Read the model definition and answer for the solid it produces. Units are mm, in the model's axes. Face numbers are marked on the shaded views. A direction names the side the tool comes from. Round coordinates to 2 decimals unless told otherwise and drop trailing zeros. Loops run counter-clockwise (first coordinate to the right, second up) from the corner with the lowest first, then second, coordinate; pieces in that order, holes last. Notation, with made-up numbers: M 50,52.25 L 76,52.25 A18 cw 76,78.25 Z; hole C 59,-27.5 d8. An arc over 180 degrees is marked long. Write each question's results on one line, items separated by ' | '.
from build123d import *
from OCP.BRepFilletAPI import BRepFilletAPI_MakeChamfer

# Parameters (mm, degrees)
ESQUISSE1_W             = 20
ESQUISSE1_H             = 34
BOSS_EXTRU_1_DEPTH      = 4
ESQUISSE2_W             = 8
ESQUISSE2_H             = 7
ENL_V_MAT_EXTRU_1_DEPTH = 21.124611797
CONG_1_R                = 4
ESQUISSE3_W             = 6
ESQUISSE3_H             = 34
BOSS_EXTRU_2_DEPTH      = 20
ESQUISSE4_R             = 2.1
ENL_V_MAT_EXTRU_2_DEPTH = 36.566838488
CHANFREIN1_SIZE         = 8
CHANFREIN1_SIZE2        = 4.618802154
CONG_2_R                = 4
ESQUISSE5_R             = 3.2
ENL_V_MAT_EXTRU_3_DEPTH = 29.08914381
ESQUISSE6_R             = 5.5
ENL_V_MAT_EXTRU_4_DEPTH = 29.08914381
ENL_V_MAT_EXTRU_5_DEPTH = 36.566838488
CONG_3_R                = 4
ESQUISSE9_W             = 30.59391243
ESQUISSE9_H             = 32.996523038
ENL_V_MAT_EXTRU_6_DEPTH = 1
ESQUISSE10_R            = 4
ENL_V_MAT_EXTRU_7_DEPTH = 3


with BuildPart() as part:
    # Esquisse1 → Boss.-Extru.1 (new body)
    with BuildSketch(Plane.XY):
        Rectangle(ESQUISSE1_W, ESQUISSE1_H)
    extrude(amount=BOSS_EXTRU_1_DEPTH)

    # Esquisse2 → Enlèv. mat.-Extru.1 (cut, through all)
    with BuildSketch(Plane.XY.offset(4)):
        with Locations((0, 13.5)):
            Rectangle(ESQUISSE2_W, ESQUISSE2_H)
        with Locations((0, -13.5)):
            Rectangle(ESQUISSE2_W, ESQUISSE2_H)
    extrude(amount=-ENL_V_MAT_EXTRU_1_DEPTH, mode=Mode.SUBTRACT)

    # Congé1
    cong_1_edges = [part.edges().sort_by_distance(p)[0] for p in [
        (0, -10, 4),
        (0, 10, 4),
    ]]
    fillet(cong_1_edges, radius=CONG_1_R - 0.0001)  # a hair under: the kernel refuses the full size

    # Esquisse3 → Boss.-Extru.2 (add)
    with BuildSketch(Plane.XY.offset(4)):
        with Locations((-7, 0)):
            Rectangle(ESQUISSE3_W, ESQUISSE3_H)
        with Locations((7, 0)):
            Rectangle(ESQUISSE3_W, ESQUISSE3_H)
    extrude(amount=BOSS_EXTRU_2_DEPTH)

    # Esquisse4 → Enlèv. mat.-Extru.2 (cut, through all)
    with BuildSketch(Plane(origin=(10, 0, 0), x_dir=(0, 0, -1), z_dir=(1, 0, 0))):
        with Locations(Location((-19, 9, 0), (0, 0, 90))):
            Circle(ESQUISSE4_R)
        with Locations(Location((-19, -9, 0), (0, 0, 90))):
            Circle(ESQUISSE4_R)
    extrude(amount=-ENL_V_MAT_EXTRU_2_DEPTH, mode=Mode.SUBTRACT)

    # Chanfrein1: one chamfer whose edges measure the first distance from different faces: ONE call of the kernel's chamfer builder (chamfer() names one face for all edges)
    chanfrein1_edges_1 = [part.edges().sort_by_distance(p)[0] for p in [
        (-7, -17, 24),
    ]]
    chanfrein1_side_1 = [part.faces().sort_by_distance(p)[0] for p in [
        (-7, -17, 12),
    ]]
    chanfrein1_edges_2 = [part.edges().sort_by_distance(p)[0] for p in [
        (-7, 17, 24),
    ]]
    chanfrein1_side_2 = [part.faces().sort_by_distance(p)[0] for p in [
        (-7, 17, 12),
    ]]
    chanfrein1_edges_3 = [part.edges().sort_by_distance(p)[0] for p in [
        (7, -17, 24),
    ]]
    chanfrein1_side_3 = [part.faces().sort_by_distance(p)[0] for p in [
        (7, -17, 12),
    ]]
    chanfrein1_edges_4 = [part.edges().sort_by_distance(p)[0] for p in [
        (7, 17, 24),
    ]]
    chanfrein1_side_4 = [part.faces().sort_by_distance(p)[0] for p in [
        (7, 17, 12),
    ]]
    chanfrein1 = BRepFilletAPI_MakeChamfer(part.part.solid().wrapped)
    for e in chanfrein1_edges_1:
        chanfrein1.Add(CHANFREIN1_SIZE, CHANFREIN1_SIZE2, e.wrapped, chanfrein1_side_1[0].wrapped)  # the first distance lies on this face
    for e in chanfrein1_edges_2:
        chanfrein1.Add(CHANFREIN1_SIZE, CHANFREIN1_SIZE2, e.wrapped, chanfrein1_side_2[0].wrapped)  # the first distance lies on this face
    for e in chanfrein1_edges_3:
        chanfrein1.Add(CHANFREIN1_SIZE, CHANFREIN1_SIZE2, e.wrapped, chanfrein1_side_3[0].wrapped)  # the first distance lies on this face
    for e in chanfrein1_edges_4:
        chanfrein1.Add(CHANFREIN1_SIZE, CHANFREIN1_SIZE2, e.wrapped, chanfrein1_side_4[0].wrapped)  # the first distance lies on this face
    add(Compound.cast(chanfrein1.Shape()), mode=Mode.REPLACE)

    # Congé2
    cong_2_edges = [part.edges().sort_by_distance(p)[0] for p in [
        (-7, 12.381197846, 24),
        (-7, -12.381197846, 24),
        (-7, -17, 16),
        (7, 12.381197846, 24),
        (7, -12.381197846, 24),
        (7, -17, 16),
        (-7, 17, 16),
        (7, 17, 16),
    ]]
    fillet(cong_2_edges, radius=CONG_2_R)

    # Esquisse5 → Enlèv. mat.-Extru.3 (cut, through all)
    with BuildSketch(Plane.XY.offset(4)):
        Circle(ESQUISSE5_R)
    extrude(amount=-ENL_V_MAT_EXTRU_3_DEPTH, mode=Mode.SUBTRACT)

    # Esquisse6 → Enlèv. mat.-Extru.4 (cut, through all)
    with BuildSketch(Plane.XY.offset(4)):
        Circle(ESQUISSE6_R)
    extrude(amount=ENL_V_MAT_EXTRU_4_DEPTH, mode=Mode.SUBTRACT)

    # Esquisse8 → Enlèv. mat.-Extru.5 (cut, through all)
    with BuildSketch(Plane(origin=(10, 0, 0), x_dir=(0, 0, -1), z_dir=(1, 0, 0))):
        Polygon((0, 17), (0, 10), (-24, -3), (-24, 17), align=None)
    extrude(amount=-ENL_V_MAT_EXTRU_5_DEPTH, mode=Mode.SUBTRACT)

    # Congé3
    cong_3_edges = [part.edges().sort_by_distance(p)[0] for p in [
        (7.304886114, -3, 24),
        (-7.304886114, -3, 24),
    ]]
    fillet(cong_3_edges, radius=CONG_3_R)

    # Esquisse9 → Enlèv. mat.-Extru.6 (cut)
    with BuildSketch(Plane(origin=(10, 0, 0), x_dir=(0, 0, -1), z_dir=(1, 0, 0))):
        with Locations((-11.472185, -1.799431883)):
            Rectangle(ESQUISSE9_W, ESQUISSE9_H)
    extrude(amount=-ENL_V_MAT_EXTRU_6_DEPTH, mode=Mode.SUBTRACT)

    # Esquisse10 → Enlèv. mat.-Extru.7 (cut)
    with BuildSketch(Plane(origin=(9, 0, 0), x_dir=(0, 0, -1), z_dir=(1, 0, 0))):
        with Locations(Location((-19, -9, 0), (0, 0, 90))):
            Circle(ESQUISSE10_R)
    extrude(amount=-ENL_V_MAT_EXTRU_7_DEPTH, mode=Mode.SUBTRACT)


solid = part.part
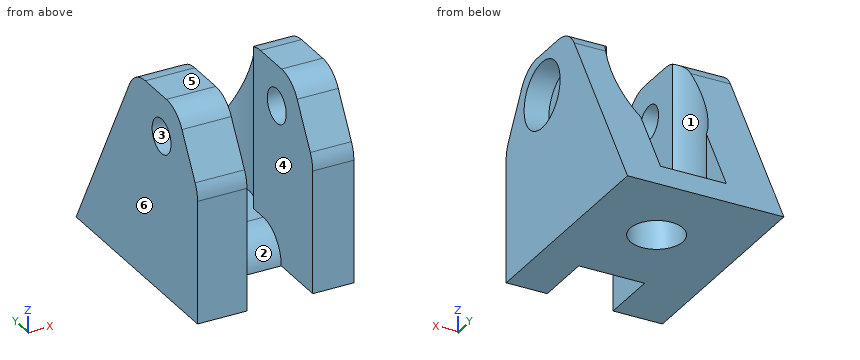
Item 1: The part is cut by section D-D (x = -7.75). Determine the outline of the cut face in (y, z).
Outcome:
outline: M -17,0 L 10,0 L -1.87,21.91 A4 ccw -5.38,24 L -10.07,24 A4 ccw -13.54,22 L -16.46,16.93 A4 ccw -17,14.93 Z; hole C -9,19 d4.2
Item 2: For the marked faces 1, 2 and 3, determine the directions among +Z, -Z, +X, -X, +Y, -Y from which every point of the face is accessible in a straight line to the end or side of a thin tool.
Outcome:
face 1: +Z | face 2: +Z, -Y | face 3: +X, -X
Item 3: Flat-ended cylindrical pins translate along their axes: pin 1 (9 mm diameter, centred on x = 2, y = -1, fed in from +Z); pin 2 (2 mm diameter, centred on x = -2, y = 2, fed in from +Z); pin 3 (5.5 mm diameter, centred on y = -9, z = 19, fed in from +X); pin 4 (5.5 mm diameter, centred on y = -9, z = 19, fed in from -X). Find the tip coordinate at first contact, or state that the pin passes through.
Outcome:
pin 1: stops at z = 23.98 | pin 2: stops at z = 4 | pin 3: stops at x = 6 | pin 4: stops at x = -10
Item 4: The part is cut by section B-B (z = 7). Determine the outline of the cut face in (x, y).
Outcome:
outline: M -10,-17 L -4,-17 L -4,-3.77 A5.5 cw -4,3.77 L -4,6.21 L -10,6.21 Z; M 4,-17 L 9,-17 L 9,6.21 L 4,6.21 L 4,3.77 A5.5 cw 4,-3.77 Z
Item 5: The part is cut by section C-C (y = -7.5). Determine the outline of the cut face in (x, z), plus the area to 3 significant figures.
Outcome:
outline: M -10,0 L 9,0 L 9,15.29 L 6,15.29 L 6,17.53 L 4,17.53 L 4,3.71 L -4,3.71 L -4,17.53 L -10,17.53 Z; M -10,20.47 L -4,20.47 L -4,24 L -10,24 Z; M 4,20.47 L 6,20.47 L 6,22.71 L 9,22.71 L 9,24 L 4,24 Z | area: 248 mm2
Item 6: The mould has two halves that part along X. Classify the marked faces 4, 5 and 6: pulls with the +X half, pulls with the -X half, needs draft (parallel to the pull), parting line crosses it, or undercut.
Outcome:
face 4: undercut | face 5: needs draft | face 6: pulls with the -X half
Item 7: Straight lines are drawn through the part: line 1 (X direction, y = -10.25, z = 1.25); line 2 (Z direction, x = 5, y = -9); line 3 (Z direction, x = 7.75, y = -9). For each, find the intervals that lie inside material, in ascending order.
Outcome:
line 1: x = -10 to -4, 4 to 9 | line 2: z = 0 to 16.9, 21.1 to 24 | line 3: z = 0 to 15, 23 to 24
